```python
from build123d import *

# Parameters (mm, degrees)
SKIZZE1_W                        = 36
SKIZZE1_H                        = 36
PLATINE_DEPTH                    = 1
F_3_2_3_2_DURCHMESSER_BOHRUNG1_D = 3.2
ANSCHLUESSE_MINUS_DEPTH          = 0.3
ANSCHLUESSE_MINUS_DEPTH_BACK     = 2.5
SKIZZE5_R                        = 1.25
SKIZZE5_R_2                      = 1
ANSCHLUESSE_PLUS_DEPTH           = 0.3
ANSCHLUESSE_PLUS_DEPTH_BACK      = 2.5
SKIZZE6_R                        = 1
SKIZZE6_R_2                      = 1.25
SKIZZE7_R                        = 1
SKUND_RANSCHL_SSE_DEPTH          = 1


with BuildPart() as part:
    # Skizze1 → Platine (new body)
    with BuildSketch(Plane(origin=(0, 0, 0), x_dir=(1, 0, 0), z_dir=(0, 1, 0))):
        Rectangle(SKIZZE1_W, SKIZZE1_H)
    extrude(amount=PLATINE_DEPTH)

    # 3.2 _3.2_ Durchmesser Bohrung1 (through all)
    with Locations(Plane(origin=(0, 1, 0), x_dir=(1, 0, 0), z_dir=(0, 1, 0))):
        with Locations((-15.25, 15.25), (15.25, 15.25), (15.25, -15.25), (-15.25, -15.25)):
            Hole(F_3_2_3_2_DURCHMESSER_BOHRUNG1_D / 2)

    # Skizze5 → Anschluesse_Minus (add, two sides: drawn at the far end of the back side and taken through both)
    with BuildSketch(Plane(origin=(18, 0, 0), x_dir=(0, 0, -1), z_dir=(1, 0, 0)).offset(-ANSCHLUESSE_MINUS_DEPTH_BACK)):
        with Locations(Location((-8, 1.5, 0), (0, 0, 203.578178478))):
            Circle(SKIZZE5_R)
        with Locations(Location((-4, 1.5, 0), (0, 0, 210))):
            Circle(SKIZZE5_R_2)
        with Locations(Location((0, 1.5, 0), (0, 0, 210))):
            Circle(SKIZZE5_R_2)
        with Locations(Location((4, 1.5, 0), (0, 0, 210))):
            Circle(SKIZZE5_R_2)
        with Locations(Location((8, 1.5, 0), (0, 0, 210))):
            Circle(SKIZZE5_R_2)
    extrude(amount=ANSCHLUESSE_MINUS_DEPTH + ANSCHLUESSE_MINUS_DEPTH_BACK)

    # Skizze6 → Anschluesse_Plus (add, two sides: drawn at the far end of the back side and taken through both)
    with BuildSketch(Plane.ZY.offset(18).offset(-ANSCHLUESSE_PLUS_DEPTH_BACK)):
        with Locations(Location((-8, 1.5, 0), (0, 0, 330))):
            Circle(SKIZZE6_R)
        with Locations(Location((-4, 1.5, 0), (0, 0, 330))):
            Circle(SKIZZE6_R)
        with Locations(Location((0, 1.5, 0), (0, 0, 330))):
            Circle(SKIZZE6_R)
        with Locations(Location((4, 1.5, 0), (0, 0, 330))):
            Circle(SKIZZE6_R)
        with Locations(Location((8, 1.5, 0), (0, 0, 336.421821522))):
            Circle(SKIZZE6_R_2)
    extrude(amount=ANSCHLUESSE_PLUS_DEPTH + ANSCHLUESSE_PLUS_DEPTH_BACK)

    # Skizze7 → Skund_ranschl_sse (add)
    with BuildSketch(Plane(origin=(0, 1, 0), x_dir=(1, 0, 0), z_dir=(0, 1, 0))):
        with Locations(Location((-9, 16.5, 0), (0, 0, 90))):
            Circle(SKIZZE7_R)
        with Locations(Location((-5, 16.5, 0), (0, 0, 90))):
            Circle(SKIZZE7_R)
        with Locations(Location((5, 16.5, 0), (0, 0, 90))):
            Circle(SKIZZE7_R)
        with Locations(Location((9, 16.5, 0), (0, 0, 90))):
            Circle(SKIZZE7_R)
        with Locations(Location((3, -13, 0), (0, 0, 90))):
            Circle(SKIZZE7_R)
        with Locations(Location((7, -13, 0), (0, 0, 90))):
            Circle(SKIZZE7_R)
    extrude(amount=SKUND_RANSCHL_SSE_DEPTH)


solid = part.part
```
The model under review builds one solid part; all positions refer to its coordinate system, in mm. A direction names the side the tool comes from. Round coordinates to 2 decimals unless told otherwise and drop trailing zeros. Write each loop counter-clockwise with the first axis right and the second up, starting at its lowest first coordinate (ties: lowest second). Pieces come first, ordered by that corner, then holes. Notation, with made-up numbers: (6, -3.75) -> (51, -3.75) arc R34 ccw to (51, 31.25) -> close; hole circle Ø7 at (29.25, 50). An arc over 180 degrees is marked (long way). Use CSV: the item, a comma, the result in double quotes.
Q1. For pin 1 Ø2.5 at (x, z) = (-15.25, -15.25) entering from -Y; pin 2 Ø11 at (x, z) = (0, 4.5) entering from +Y; pin 3 Ø0.6 at (x, z) = (-5, -16) entering from +Y; pin 4 Ø1.5 at (y, z) = (1, 10) entering from +X, all flat-tipped, find the tip position at first contact; note any pin that passes through.
Checks:
pin 1,"through"
pin 2,"y = 1"
pin 3,"y = 2"
pin 4,"x = 18"
Q2. To check wall thickness, follow probe 1 along X at (y, z) = (0.65, 15.25); probe 2 along Y at (x, z) = (-14, -10). State the ranges of each line that lie inside material, in increasing order. Write a range as [from, to].
Checks:
probe 1,"[-18, -16.85], [-13.65, 13.65], [16.85, 18]"
probe 2,"[0, 1]"
Q3. For faces 1 (the flat face through (-15.5, 2, -4)), 2 (the cylindrical face through (-5.3, 1.493, -17.454)), 3 (the cylindrical face through (16.43, 0.49, 14.17)), list the 3-axis set-ups (+Z, -Z, +X, -X, +Y, -Y) from which the entire face can be reached by the end or side of a thin tool; tool diameter is ignored.
Checks:
face 1,"+Z, -Z, +Y"
face 2,"+Y"
face 3,"+Y, -Y"
Q4. Consider section B-B (y = 1.5). State how many separate pieces and enclosed holes the cut face has, then the cut area to 3 significant figures.
Checks:
separate pieces,"16"
enclosed holes,"0"
area,"77.6 mm²"
Q5. Mouldability with a two-part tool opening along X and no side actions: class faces 4 (the flat face through (18, 0.3, 0.3)), 5 (the cylindrical face through (3.383, 1.493, 12.076)), 6 (the flat face through (-0.3, 0.5, 18)) as released by +X, released by -X, zero draft, split by the parting line, or undercut.
Checks:
face 4,"released by +X"
face 5,"undercut"
face 6,"zero draft"
Q6. Consider section D-D (z = -4). Give the boundary of the cut face in (x, y), then the cut area to 3 significant figures.
Checks:
outline,"(-18.3, 0.5) -> (-18, 0.5) -> (-18, 0) -> (18, 0) -> (18, 0.5) -> (18.3, 0.5) -> (18.3, 2.5) -> (15.5, 2.5) -> (15.5, 1) -> (-15.5, 1) -> (-15.5, 2.5) -> (-18.3, 2.5) -> close"
area,"44.7 mm²"
Q7. Consider section C-C (x = 7). Give the boundary of the cut face in (y, z), then the cut area to 3 significant figures.
Checks:
outline,"(0, -18) -> (1, -18) -> (1, 12) -> (2, 12) -> (2, 14) -> (1, 14) -> (1, 18) -> (0, 18) -> close"
area,"38.0 mm²"
Q8. Consider section A-A (z = 15.25). Give the boundary of the cut face in (x, y).
Checks:
outline,"(-18, 0) -> (-16.85, 0) -> (-16.85, 1) -> (-18, 1) -> close; (-13.65, 0) -> (13.65, 0) -> (13.65, 1) -> (-13.65, 1) -> close; (16.85, 0) -> (18, 0) -> (18, 1) -> (16.85, 1) -> close"
